```python
from build123d import *

# Parameters (mm, degrees)
SKETCH1_R           = 45
SKETCH1_R_2         = 42
BOSS_EXTRUDE1_DEPTH = 15
BOSS_EXTRUDE2_START = -15
SKETCH1_3_R         = 10
SKETCH1_3_R_2       = 3
BOSS_EXTRUDE2_DEPTH = 15
BOSS_EXTRUDE3_START = -5
SKETCH2_W           = 14
SKETCH2_H           = 37.310793113
BOSS_EXTRUDE3_DEPTH = 17
CIRPATTERN1_COUNT   = 3
SKETCH1_4_R         = 50
SKETCH1_4_R_2       = 45
BOSS_EXTRUDE4_DEPTH = 13


with BuildPart() as part:
    # Sketch1 → Boss-Extrude1 (new body, symmetric)
    with BuildSketch(Plane.XY):
        Circle(SKETCH1_R)
        Circle(SKETCH1_R_2, mode=Mode.SUBTRACT)
    extrude(amount=BOSS_EXTRUDE1_DEPTH, both=True)



with BuildPart() as body_2:
    # Sketch1<3> → Boss-Extrude2 (new body)
    with BuildSketch(Plane.XY.offset(BOSS_EXTRUDE2_START)):
        Circle(SKETCH1_3_R)
        Circle(SKETCH1_3_R_2, mode=Mode.SUBTRACT)
    extrude(amount=BOSS_EXTRUDE2_DEPTH)


with BuildPart() as part_1:
    add(part.part)

    add(body_2.part)  # Boss-Extrude3 merges body 2
    # Sketch2 → Boss-Extrude3 (add)
    with BuildSketch(Plane.XY.offset(BOSS_EXTRUDE3_START)):
        with Locations((0, 25.796824986)):
            Rectangle(SKETCH2_W, SKETCH2_H)
        with BuildLine():
            Line((1.5, 36), (1.5, 16))
            ThreePointArc((1.5, 16), (0, 14.5), (-1.5, 16))
            Line((-1.5, 16), (-1.5, 36))
            ThreePointArc((-1.5, 36), (0, 37.5), (1.5, 36))
        make_face(mode=Mode.SUBTRACT)
    boss_extrude3 = extrude(amount=BOSS_EXTRUDE3_DEPTH)

    # CirPattern1: Boss-Extrude3 ×3 about axis
    cirpattern1_axis = Axis((0, 0, 0), (0, 0, 1))
    for i in range(1, CIRPATTERN1_COUNT):
        add(boss_extrude3.rotate(cirpattern1_axis, i * 360 / CIRPATTERN1_COUNT))

    # Sketch3 → Cut-Revolve1 (revolve, cut)
    with BuildSketch(Plane(origin=(0, 0, 0), x_dir=(0, 0, -1), z_dir=(1, 0, 0))):
        Polygon((0, 0), (0, -10), (-15, -42), (-15, 0), align=None)
        Polygon((4.969855419, -10), (15, -10), (15, -42), (-10.030144581, -42), align=None)
    revolve(axis=Axis((0, 0, 0), (0, 0, 1)), mode=Mode.SUBTRACT)

    # Sketch1<4> → Boss-Extrude4 (add, symmetric)
    with BuildSketch(Plane.XY):
        Circle(SKETCH1_4_R)
        Circle(SKETCH1_4_R_2, mode=Mode.SUBTRACT)
    extrude(amount=BOSS_EXTRUDE4_DEPTH, both=True)


solid = part_1.part
```
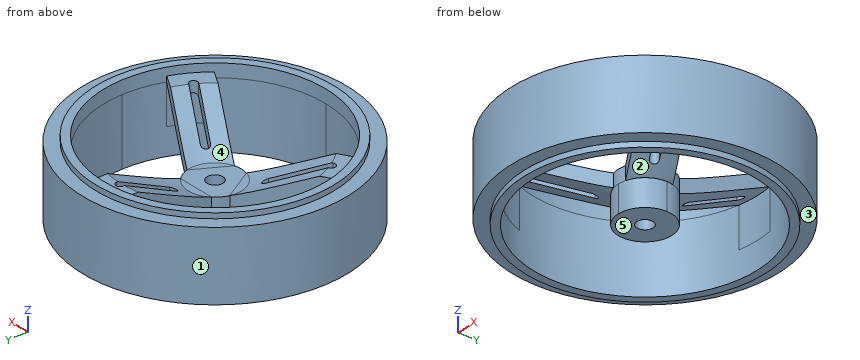
Part model, mm, in its own coordinate system. Face numbers are marked on the shaded views. A direction names the side the tool comes from. Round coordinates to 2 decimals unless told otherwise and drop trailing zeros. Loops run counter-clockwise (first coordinate to the right, second up) from the corner with the lowest first, then second, coordinate; pieces in that order, holes last. Notation, with made-up numbers: (20, 37.25) -> (71, 37.25) arc R14 ccw to (71, 61.25) -> close; hole circle Ø1 at (36, 34). An arc over 180 degrees is marked (long way). Use CSV: the item, a comma, the result in double quotes. Start each with the question number.
1) Cut at A-A, the plane z = -6.75. Write the cut outline in (x, y).
2) Drop flat-ended pins along their axis: P1, Ø6.5, axis at x = 35.5, y = -22, coming from the +Z side; P2, Ø8, axis at x = 16, z = 11.5, coming from the +Y side; P3, Ø6, axis at x = 18, z = -10, coming from the -Y side; P4, Ø8.5, axis at y = 25, z = 4, coming from the +X side. Give the stop position or say it passes through.
3) Cut at B-B, the plane z = 5.75. Write the cut outline in (x, y) (3 decimals), plus the area to 3 significant figures.
4) Wall check: L1, parallel to Y at x = 0, z = -7.5; L2, parallel to Y at x = 0, z = 4.75; L3, parallel to Y at x = 13, z = -9.25. Give the ranges that are in metal, low to high. Write a range as [from, to].
5) Pull direction X, two halves, no side cores. Call the marked faces 1, 2 and 3: +X half, -X half, draft (parallel to the pull), parting line (faces both ways), or undercut.
6) Which spindle directions (+Z, -Z, +X, -X, +Y, -Y) get a long thin tool onto all of the face, cutting with end or side? Do the marked faces 4 and 5. Say none if no direction does.
7) Cut at C-C, the plane x = 23. Give the number of separate pieces and of enclosed holes in the cut face, plus the area to 3 significant figures.
Determined:
1,outline,"circle Ø100 at (0, 0); circle Ø20 at (0, 0); hole circle Ø84 at (0, 0); hole circle Ø6 at (0, 0)"
2,P1,"stops at z = 15"
2,P2,"stops at y = 48.54"
2,P3,"stops at y = -47.7"
2,P4,"stops at x = 45.49"
3,outline,"circle Ø100 at (0, 0); (-31.312, -9.995) arc R32.869 ccw to (-29.186, -15.118) -> (-19.99, -9.809) arc R22.267 cw to (-21.806, -4.507) -> close; (-27.686, -17.716) arc R32.869 ccw to (-24.312, -22.12) -> (-14.806, -16.631) arc R22.267 cw to (-18.49, -12.407) -> close; (-7, 21.138) arc R22.267 cw to (-1.5, 22.216) -> (-1.5, 32.835) arc R32.869 ccw to (-7, 32.115) -> close; (1.5, 22.216) arc R22.267 cw to (7, 21.138) -> (7, 32.115) arc R32.869 ccw to (1.5, 32.835) -> close; (14.806, -16.631) -> (24.312, -22.12) arc R32.869 ccw to (27.686, -17.716) -> (18.49, -12.407) arc R22.267 cw to start; (19.99, -9.809) -> (29.186, -15.118) arc R32.869 ccw to (31.312, -9.995) -> (21.806, -4.507) arc R22.267 cw to start; hole circle Ø84 at (0, 0)"
3,area,"2,670 mm2"
4,L1,"y = [-50, -42], [-10, -3], [3, 10], [42, 50]"
4,L2,"y = [-50, -42], [42, 50]"
4,L3,"y = [-48.28, -39.94], [39.94, 48.28]"
5,face 1,"parting line"
5,face 2,"undercut"
5,face 3,"draft"
6,face 4,"+Z"
6,face 5,"-Z, +X, -X, +Y, -Y"
7,separate pieces,"4"
7,enclosed holes,"0"
7,area,"573 mm2"
